```python
from build123d import *

# Parameters (mm, degrees)
F0_W     = 2
F0_H     = 22.5
F0_W_2   = 55
F0_H_2   = 18
F1_DEPTH = 4
F0_W_3   = 25
F0_H_3   = 12
F2_DEPTH = 20
F3_DEPTH = 40


with BuildPart() as f1:
    # F0 (on Top) → F1 (new body)
    with BuildSketch(Plane.XY):
        with BuildLine():
            Line((54.401939, 14.236366), (-46.598061, 14.236366))
            ThreePointArc((-46.598061, 14.236366), (-50.133595, 12.7719), (-51.598061, 9.236366))
            Line((-51.598061, 9.236366), (-51.598061, -13.263634))
            ThreePointArc((-51.598061, -13.263634), (-50.133595, -16.799168), (-46.598061, -18.263634))
            Line((-46.598061, -18.263634), (54.401939, -18.263634))
            ThreePointArc((54.401939, -18.263634), (57.937472, -16.799168), (59.401939, -13.263634))
            Line((59.401939, -13.263634), (59.401939, 9.236366))
            ThreePointArc((59.401939, 9.236366), (57.937472, 12.7719), (54.401939, 14.236366))
        make_face()
        with Locations((-49.348061, -2.013634)):
            Rectangle(F0_W, F0_H, mode=Mode.SUBTRACT)
        with Locations((-13.098061, -0.263634)):
            Rectangle(F0_W_2, F0_H_2, mode=Mode.SUBTRACT)
        with BuildLine():
            Line((54.401939, -11.263634), (45.401939, -11.263634))
            Line((45.401939, -11.263634), (45.401939, -14.263634))
            Line((45.401939, -14.263634), (18.901939, -14.263634))
            Line((18.901939, -14.263634), (17.401939, -14.263634))
            Line((17.401939, -14.263634), (17.401939, 3.736366))
            Line((17.401939, 3.736366), (29.901939, 3.736366))
            Line((29.901939, 3.736366), (29.901939, 12.736366))
            Line((29.901939, 12.736366), (43.901939, 12.736366))
            Line((43.901939, 12.736366), (43.901939, 3.736366))
            Line((43.901939, 3.736366), (45.401939, 3.736366))
            Line((45.401939, 3.736366), (45.401939, 0.736366))
            Line((45.401939, 0.736366), (45.401939, -3.763634))
            ThreePointArc((45.401939, -3.763634), (46.719958, -0.581654), (49.901939, 0.736366))
            ThreePointArc((49.901939, 0.736366), (53.083919, -0.581654), (54.401939, -3.763634))
            Line((54.401939, -3.763634), (54.401939, -11.263634))
        make_face(mode=Mode.SUBTRACT)
        with Locations((57.151939, -2.013634)):
            Rectangle(F0_W, F0_H, mode=Mode.SUBTRACT)
    extrude(amount=F1_DEPTH)

    # F0 (on Top) → F2 (join)
    with BuildSketch(Plane.XY):
        Polygon((45.401939, -14.263634), (45.401939, -11.263634), (45.401939, -3.763634), (45.401939, 0.736366), (45.401939, 3.736366), (43.901939, 3.736366), (29.901939, 3.736366), (17.401939, 3.736366), (17.401939, -14.263634), (18.901939, -14.263634), align=None)
        with Locations((31.401939, -5.263634)):
            Rectangle(F0_W_3, F0_H_3, mode=Mode.SUBTRACT)
    extrude(amount=F2_DEPTH)

    # F0 (on Top) → F3 (join)
    with BuildSketch(Plane.XY):
        with Locations((57.151939, -2.013634)):
            Rectangle(F0_W, F0_H)
        with Locations((-49.348061, -2.013634)):
            Rectangle(F0_W, F0_H)
    extrude(amount=F3_DEPTH)


solid = f1.part
```
Source: CAD feature listing. Evaluate the final solid. Frame: model axes, mm. A direction names the side the tool comes from. Give positions to 0.01 mm unless a question says otherwise; leave off trailing zeros. Write each loop counter-clockwise with the first axis right and the second up, starting at its lowest first coordinate (ties: lowest second). Pieces come first, ordered by that corner, then holes.
1. Section query A-A (x = 27.5). Return the cut outline in (y, z).
2. Pull-direction query (X, two-part tool) for faces 1 (the face through (45.402, -5, 12)), 2 (the face through (3, 9, 0)), 3 (the face through (57.98, 12.73, 1.97)); classes: +X half, -X half, draft (parallel to the pull), parting line (faces both ways), or undercut.
3. Access query for faces 4 (the face through (57, -13.264, 22)), 5 (the face through (-49, 9.236, 22)), 6 (the face through (50, -11.264, 2)). Directions: +Z, -Z, +X, -X, +Y, -Y. A direction counts if a zero-diameter tool reaches every point of the face in a straight line with its end or side. Return the directions, or none.
4. Section query D-D (y = -5). Return the cut outline in (x, z).
5. Section query B-B (y = 7). Return the cut outline in (x, z), then the cut area to 3 significant figures.
6. First-contact query: pin 1 (18 mm diameter, centred on y = -6.5, z = 19.5, fed in from -X); pin 2 (13 mm diameter, centred on x = 26.5, z = 11.5, fed in from -Y); pin 3 (4 mm diameter, centred on y = -0.5, z = 10.5, fed in from +X); pin 4 (8 mm diameter, centred on x = -5, z = 11, fed in from +Y). Flat tips, straight axial feed; report the tip coordinate or a pass-through.
7. Section query C-C (z = 9). Return the cut outline in (x, y), then the cut area to 3 significant figures.
8. Material intervals for line 1 along X through (y, z) = (-12, 19.5); line 2 along X through (y, z) = (-1, 12.5); line 3 along X through (y, z) = (-11, 36.5), sorted ascending.
Output values:
1. outline: (-18.26, 0) - (-11.26, 0) - (-11.26, 20) - (-14.26, 20) - (-14.26, 4) - (-18.26, 4) - close; (0.74, 0) - (14.24, 0) - (14.24, 4) - (3.74, 4) - (3.74, 20) - (0.74, 20) - close
2. face 1: undercut
2. face 2: draft
2. face 3: +X half
3. face 4: +Z, +X, -Y
3. face 5: +Z, +X, -X, +Y
3. face 6: +Z, -Z
4. outline: (-51.6, 0) - (-40.6, 0) - (-40.6, 4) - (-48.35, 4) - (-48.35, 40) - (-50.35, 40) - (-50.35, 4) - (-51.6, 4) - close; (14.4, 0) - (18.9, 0) - (18.9, 20) - (17.4, 20) - (17.4, 4) - (14.4, 4) - close; (43.9, 0) - (45.4, 0) - (45.4, 20) - (43.9, 20) - close; (54.4, 0) - (59.4, 0) - (59.4, 4) - (58.15, 4) - (58.15, 40) - (56.15, 40) - (56.15, 4) - (54.4, 4) - close
5. outline: (-51.6, 0) - (-40.6, 0) - (-40.6, 4) - (-48.35, 4) - (-48.35, 40) - (-50.35, 40) - (-50.35, 4) - (-51.6, 4) - close; (14.4, 0) - (29.9, 0) - (29.9, 4) - (14.4, 4) - close; (43.9, 0) - (59.4, 0) - (59.4, 4) - (58.15, 4) - (58.15, 40) - (56.15, 40) - (56.15, 4) - (43.9, 4) - close
5. area: 312 mm2
6. pin 1: stops at x = -50.35
6. pin 2: stops at y = -14.26
6. pin 3: stops at x = 58.15
6. pin 4: passes through
7. outline: (-50.35, -13.26) - (-48.35, -13.26) - (-48.35, 9.24) - (-50.35, 9.24) - close; (17.4, -14.26) - (45.4, -14.26) - (45.4, 3.74) - (17.4, 3.74) - close; (56.15, -13.26) - (58.15, -13.26) - (58.15, 9.24) - (56.15, 9.24) - close; hole (18.9, -11.26) - (43.9, -11.26) - (43.9, 0.74) - (18.9, 0.74) - close
7. area: 294 mm2
8. line 1: x = -50.35 to -48.35, 17.4 to 45.4, 56.15 to 58.15
8. line 2: x = -50.35 to -48.35, 17.4 to 18.9, 43.9 to 45.4, 56.15 to 58.15
8. line 3: x = -50.35 to -48.35, 56.15 to 58.15
